The drawing under review shows one solid part. Ordinate dimensions are in mm from its lowest x, y, z. Give positions to 0.01 mm unless a question says otherwise; leave off trailing zeros. Write each loop counter-clockwise with the first axis right and the second up, starting at its lowest first coordinate (ties: lowest second). Pieces come first, ordered by that corner, then holes.
Q1. We need section D-D (y = 20). Write out the cut boundary in (x, z).
Q2. Mouldability with a two-part tool opening along Y and no side actions: class the marked faces 1, 2 and 3 as released by +Y, released by -Y, zero draft, split by the parting line, or undercut.
Q3. We need section B-B (z = 1.9). Give the number of separate pieces and of enclosed holes in the cut face, then the cut area to 3 significant figures.
Q4. Insertion check: P1, Ø2, axis at x = 32.5, z = 4, coming from the +Y side; P2, Ø12.5, axis at x = 19, y = 20, coming from the +Z side. Each pin has a flat end and moves straight along its axis. Give the tip position at first contact, or say it passes through.
Q5. We need section A-A (y = 58.1). Write out the cut boundary in (x, z).
Q6. For line 1 (Y direction, x = 16, z = 3.55) (1 decimal); line 2 (Y direction, x = 23, z = 2.95) (1 decimal); line 3 (X direction, y = 61.5, z = 2.7), list the stretches that pass through material, from the lowest coordinate up.
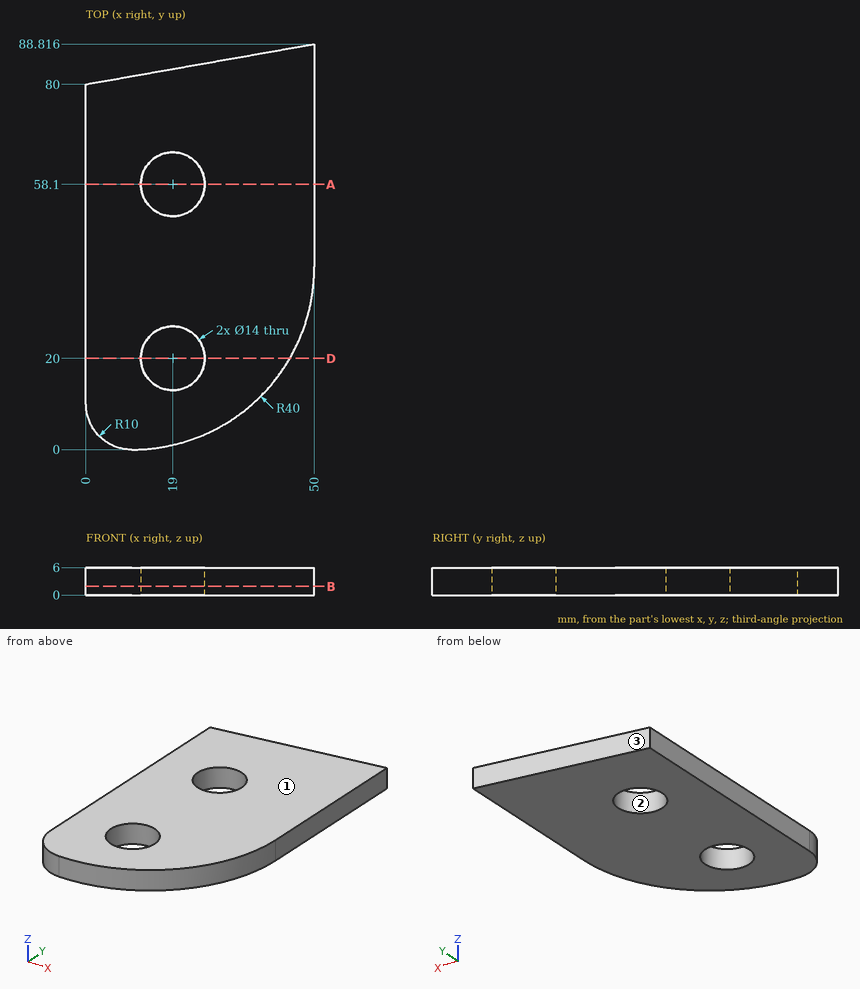
Computed:
1. outline: (0, 0) - (12, 0) - (12, 6) - (0, 6) - close; (26, 0) - (44.64, 0) - (44.64, 6) - (26, 6) - close
2. face 1: zero draft
2. face 2: undercut
2. face 3: released by +Y
3. separate pieces: 1
3. enclosed holes: 2
3. area: 3,550 mm2
4. P1: stops at y = 85.91
4. P2: passes through
5. outline: (0, 0) - (12, 0) - (12, 6) - (0, 6) - close; (26, 0) - (50, 0) - (50, 6) - (26, 6) - close
6. line 1: y = 0.5 to 13.7, 26.3 to 51.8, 64.4 to 82.8
6. line 2: y = 2.2 to 14.3, 25.7 to 52.4, 63.8 to 84.1
6. line 3: x = 0 to 12.88, 25.12 to 50
